from build123d import *

# Parameters (mm, degrees)
SKIZZE1_W                       = 300
SKIZZE1_H                       = 50
AUFSATZ_LINEAR_AUSTRAGEN1_DEPTH = 4
SKIZZE2_W                       = 15.5
SKIZZE2_H                       = 4
AUFSATZ_LINEAR_AUSTRAGEN3_DEPTH = 4
SCHNITT_LINEAR_AUSTRAGEN1_REACH = 6
SKIZZE3_W                       = 4
SKIZZE3_H                       = 17.45
SKIZZE3_H_2                     = 17.05
SKIZZE4_W                       = 50.3
SKIZZE4_H                       = 13
AUFSATZ_LINEAR_AUSTRAGEN4_DEPTH = 4
SCHNITT_LINEAR_AUSTRAGEN2_REACH = 6


with BuildPart() as part:
    # Skizze1 → Aufsatz-Linear austragen1 (new body)
    with BuildSketch(Plane.XY):
        with Locations((150, 25)):
            Rectangle(SKIZZE1_W, SKIZZE1_H)
    extrude(amount=AUFSATZ_LINEAR_AUSTRAGEN1_DEPTH)

    # Skizze2 → Aufsatz-Linear austragen3 (add)
    with BuildSketch(Plane.XY):
        with Locations((25.2, -2)):
            Rectangle(SKIZZE2_W, SKIZZE2_H)
        with Locations((75.2, -2)):
            Rectangle(SKIZZE2_W, SKIZZE2_H)
        with Locations((125.2, -2)):
            Rectangle(SKIZZE2_W, SKIZZE2_H)
        with Locations((175.2, -2)):
            Rectangle(SKIZZE2_W, SKIZZE2_H)
        with Locations((225.2, -2)):
            Rectangle(SKIZZE2_W, SKIZZE2_H)
        with Locations((275.2, -2)):
            Rectangle(SKIZZE2_W, SKIZZE2_H)
    extrude(amount=AUFSATZ_LINEAR_AUSTRAGEN3_DEPTH)

    # Skizze3 → Schnitt-Linear austragen1 (cut, up to next)
    with BuildSketch(Plane.XY.offset(4), mode=Mode.PRIVATE) as schnitt_linear_austragen1_sk1:
        with Locations((2, 41.275)):
            Rectangle(SKIZZE3_W, SKIZZE3_H)
    schnitt_linear_austragen1_tool1 = extrude(schnitt_linear_austragen1_sk1.sketch, amount=-SCHNITT_LINEAR_AUSTRAGEN1_REACH, mode=Mode.PRIVATE) & part.part
    add(schnitt_linear_austragen1_tool1.solids().sort_by_distance((2, 41.275, 4))[0], mode=Mode.SUBTRACT)
    # Skizze3 → Schnitt-Linear austragen1 (cut, up to next)
    with BuildSketch(Plane.XY.offset(4), mode=Mode.PRIVATE) as schnitt_linear_austragen1_sk2:
        with Locations((2, 8.525)):
            Rectangle(SKIZZE3_W, SKIZZE3_H_2)
    schnitt_linear_austragen1_tool2 = extrude(schnitt_linear_austragen1_sk2.sketch, amount=-SCHNITT_LINEAR_AUSTRAGEN1_REACH, mode=Mode.PRIVATE) & part.part
    add(schnitt_linear_austragen1_tool2.solids().sort_by_distance((2, 8.525, 4))[0], mode=Mode.SUBTRACT)
    # Skizze3 → Schnitt-Linear austragen1 (cut, up to next)
    with BuildSketch(Plane.XY.offset(4), mode=Mode.PRIVATE) as schnitt_linear_austragen1_sk3:
        with Locations((298, 8.525)):
            Rectangle(SKIZZE3_W, SKIZZE3_H_2)
    schnitt_linear_austragen1_tool3 = extrude(schnitt_linear_austragen1_sk3.sketch, amount=-SCHNITT_LINEAR_AUSTRAGEN1_REACH, mode=Mode.PRIVATE) & part.part
    add(schnitt_linear_austragen1_tool3.solids().sort_by_distance((298, 8.525, 4))[0], mode=Mode.SUBTRACT)
    # Skizze3 → Schnitt-Linear austragen1 (cut, up to next)
    with BuildSketch(Plane.XY.offset(4), mode=Mode.PRIVATE) as schnitt_linear_austragen1_sk4:
        with Locations((298, 41.275)):
            Rectangle(SKIZZE3_W, SKIZZE3_H)
    schnitt_linear_austragen1_tool4 = extrude(schnitt_linear_austragen1_sk4.sketch, amount=-SCHNITT_LINEAR_AUSTRAGEN1_REACH, mode=Mode.PRIVATE) & part.part
    add(schnitt_linear_austragen1_tool4.solids().sort_by_distance((298, 41.275, 4))[0], mode=Mode.SUBTRACT)

    # Skizze4 → Aufsatz-Linear austragen4 (add)
    with BuildSketch(Plane.XY.offset(4)):
        with Locations((74.15, 56.5)):
            Rectangle(SKIZZE4_W, SKIZZE4_H)
        with Locations((225.85, 56.5)):
            Rectangle(SKIZZE4_W, SKIZZE4_H)
    extrude(amount=-AUFSATZ_LINEAR_AUSTRAGEN4_DEPTH)

    # Skizze5 → Schnitt-Linear austragen2 (cut, up to next)
    with BuildSketch(Plane(origin=(0, 0, 0), x_dir=(-1, 0, 0), z_dir=(0, 0, -1)), mode=Mode.PRIVATE) as schnitt_linear_austragen2_sk1:
        Polygon((-267.589208013, 50), (-267.589208013, 32.5), (-263.589208013, 32.5), (-263.589208013, 17.5), (-267.589208013, 17.5), (-267.589208013, 0), (-260.181086132, 0), (-260.181086132, -8.903305995), (-305.118419692, -8.903305995), (-305.118419692, 50), align=None)
    schnitt_linear_austragen2_tool1 = extrude(schnitt_linear_austragen2_sk1.sketch, amount=-SCHNITT_LINEAR_AUSTRAGEN2_REACH, mode=Mode.PRIVATE) & part.part
    add(schnitt_linear_austragen2_tool1.solids().sort_by_distance((285.186351, 19.956954, 0))[0], mode=Mode.SUBTRACT)


solid = part.part
Work out the finished part from the listing and answer in its coordinate system (mm). Give positions to 0.01 mm unless a question says otherwise; leave off trailing zeros. Loops run counter-clockwise (first coordinate to the right, second up) from the corner with the lowest first, then second, coordinate; pieces in that order, holes last. Notation, with made-up numbers: M 35.25,72 L 74.25,72 A8 cw 74.25,77 Z; hole C 24,72.25 d2. An arc over 180 degrees is marked long. Use CSV: the item, a comma, the result in double quotes.
1) Given P1, Ø1.2, axis at y = 4.5, z = 2.5, coming from the -X side; P2, Ø2, axis at y = -1.5, z = 1, coming from the +X side; P3, Ø2, axis at y = 55, z = 1, coming from the +X side, each flat-ended and moving along its own axis, determine where each tip first touches the part or whether it passes through.
Answer:
P1,"x = 4"
P2,"x = 232.95"
P3,"x = 251"
2) Consider L1, parallel to X at y = 58.5, z = 1.55; L2, parallel to X at y = 44, z = 2.1; L3, parallel to X at y = 24, z = 1.95. Determine where each line is inside the solid, lowest interval first.
Answer:
L1,"49 to 99.3, 200.7 to 251"
L2,"4 to 267.59"
L3,"0 to 263.59"
3) Find section B-B on x = 46. Write down the section's boundary in (y, z).
Answer:
outline,"M 0,0 L 50,0 L 50,4 L 0,4 Z"
4) Find section C-C on x = 213. Write down the section's boundary in (y, z), plus the area to 3 significant figures.
Answer:
outline,"M 0,0 L 63,0 L 63,4 L 0,4 Z"
area,"252 mm^2"
5) Find section A-A on y = 53. Write down the section's boundary in (x, z).
Answer:
outline,"M 49,0 L 99.3,0 L 99.3,4 L 49,4 Z; M 200.7,0 L 251,0 L 251,4 L 200.7,4 Z"
